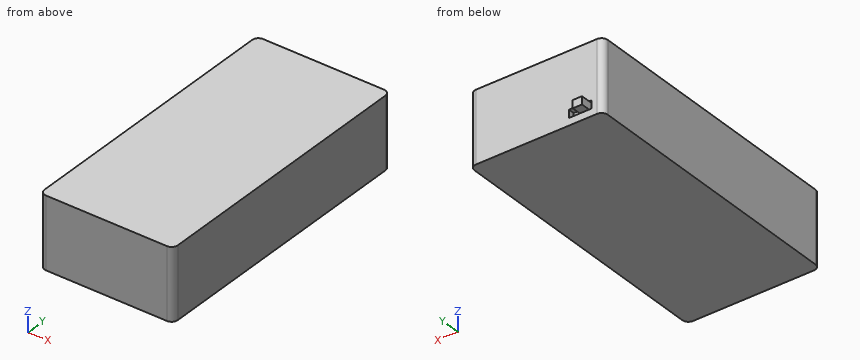
```python
from build123d import *

# Parameters (mm, degrees)
BOSS_EXTRUDE1_DEPTH = 23
SKETCH2_W           = 7.233654816
SKETCH2_H           = 2.549566861
CUT_EXTRUDE1_DEPTH  = 2
SKETCH3_W           = 3
SKETCH3_H           = 2.549566861
BOSS_EXTRUDE2_DEPTH = 5


with BuildPart() as part:
    # Sketch1 → Boss-Extrude1 (new body)
    with BuildSketch(Plane.XY):
        with BuildLine():
            Line((2, 0), (41, 0))
            ThreePointArc((41, 0), (42.414213562, 0.585786438), (43, 2))
            Line((43, 2), (43, 90))
            ThreePointArc((43, 90), (42.414213562, 91.414213562), (41, 92))
            Line((41, 92), (2, 92))
            ThreePointArc((2, 92), (0.585786438, 91.414213562), (0, 90))
            Line((0, 90), (0, 2))
            ThreePointArc((0, 2), (0.585786438, 0.585786438), (2, 0))
        make_face()
    extrude(amount=BOSS_EXTRUDE1_DEPTH)

    # Sketch2 → Cut-Extrude1 (cut)
    with BuildSketch(Plane(origin=(0, 92, 0), x_dir=(1, 0, 0), z_dir=(0, 1, 0))):
        with Locations((7.388443885, -3.61721714)):
            Rectangle(SKETCH2_W, SKETCH2_H)
    extrude(amount=-CUT_EXTRUDE1_DEPTH, mode=Mode.SUBTRACT)

    # Sketch3 → Boss-Extrude2 (add)
    with BuildSketch(Plane(origin=(0, 90, 0), x_dir=(1, 0, 0), z_dir=(0, 1, 0))):
        with Locations((6.019667475, -3.61721714)):
            Rectangle(SKETCH3_W, SKETCH3_H)
    extrude(amount=BOSS_EXTRUDE2_DEPTH)


solid = part.part
```
The model under review builds one solid part; all positions refer to its coordinate system, in mm. Coordinates: 2 decimals unless noted, no trailing zeros. Order: outer loops, then holes, each group sorted by start corner. A loop starts at its lowest first (then second) coordinate and runs counter-clockwise, first axis right, second up. Notation, with made-up numbers: M 10.25,-30.5 L 69.25,-30.5 A20 ccw 69.25,-19.5 Z; hole C 51,57 d8. An arc over 180 degrees is marked long. One line per question, with ' | ' between items.
(1) Insertion check: pin 1 (1.5 mm diameter, centred on x = 22, z = 19.5, fed in from +Y); pin 2 (0.9 mm diameter, centred on x = 6, y = 93, fed in from +Z); pin 3 (1.6 mm diameter, centred on y = 91, z = 4, fed in from -X). Each pin has a flat end and moves straight along its axis. Give the tip position at first contact, or say it passes through.
Geometry results:
pin 1: stops at y = 92 | pin 2: stops at z = 4.89 | pin 3: stops at x = 0.01
(2) For probe 1 along Y at (x, z) = (17, 5), list the stretches that pass through material, from the lowest coordinate up. Write a range as from..to.
Geometry results:
probe 1: y = 0..92
(3) Add section C-C, the plane x = 26.5. Write out the cut boundary in (y, z), then the cut area to 3 significant figures.
Geometry results:
outline: M 0,0 L 92,0 L 92,23 L 0,23 Z | area: 2,120 mm²
(4) Add section A-A, the plane x = 5.5. Write out the cut boundary in (y, z), then the cut area to 3 significant figures.
Geometry results:
outline: M 0,0 L 92,0 L 92,2.34 L 95,2.34 L 95,4.89 L 92,4.89 L 92,23 L 0,23 Z | area: 2,120 mm²
(5) Add section B-B, the plane z = 10.25. Write out the cut boundary in (x, y).
Geometry results:
outline: M 0,2 A2 ccw 2,0 L 41,0 A2 ccw 43,2 L 43,90 A2 ccw 41,92 L 2,92 A2 ccw 0,90 Z
